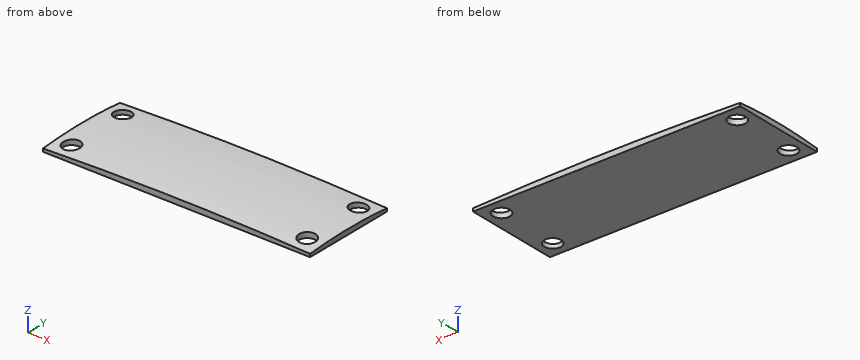
from build123d import *

# Parameters (mm, degrees)
SKETCH1_OUTSIDE_W       = 3552.458
SKETCH1_OUTSIDE_H       = 1860.818
SKETCH1_OUTSIDE_W_2     = 107.95
SKETCH1_OUTSIDE_H_2     = 38.1
CUT_EXTRUDE1_DEPTH      = 3115.745878548
CUT_EXTRUDE2_START      = -3.175
SKETCH3_W               = 107.95
SKETCH3_H               = 44.752430816
CUT_EXTRUDE2_DEPTH      = 2744.161532781
CUT_EXTRUDE3_DEPTH      = 58.326117654
CUT_EXTRUDE3_DEPTH_BACK = 58.326117654
SKETCH4_R               = 3.429


with BuildPart() as part:
    # Sketch2 → Revolve1 (revolve)
    with BuildSketch(Plane(origin=(0, 0, 0), x_dir=(0, 0, -1), z_dir=(1, 0, 0))):
        with BuildLine():
            Line((1372.87, -527.05), (1372.87, 527.05))
            add(Edge.make_bspline(
                [(1372.87, 527.05), (0, 527.05), (0, 0), (0, -527.05), (1372.87, -527.05)],
                knots=[4.71238898, 4.71238898, 4.71238898, 6.283185307, 6.283185307, 7.853981634, 7.853981634, 7.853981634], degree=2, weights=[1, 0.707106781, 1, 0.707106781, 1]))
        make_face()
    revolve(axis=Axis((0, -527.05, -1372.87), (0, 1, 0)))

    # Sketch1 outside → Cut-Extrude1 (cut, through all)
    with BuildSketch(Plane.XY):
        Rectangle(SKETCH1_OUTSIDE_W, SKETCH1_OUTSIDE_H)
        Rectangle(SKETCH1_OUTSIDE_W_2, SKETCH1_OUTSIDE_H_2, mode=Mode.SUBTRACT)
    extrude(amount=-CUT_EXTRUDE1_DEPTH, mode=Mode.SUBTRACT)

    # Sketch3 → Cut-Extrude2 (cut, through all)
    with BuildSketch(Plane.XY.offset(CUT_EXTRUDE2_START)):
        Rectangle(SKETCH3_W, SKETCH3_H)
    extrude(amount=-CUT_EXTRUDE2_DEPTH, mode=Mode.SUBTRACT)

    # Sketch4 → Cut-Extrude3 (cut, two sides: drawn at the far end of the back side and taken through both)
    with BuildSketch(Plane(origin=(0, 0, -3.175), x_dir=(-1, 0, 0), z_dir=(0, 0, -1)).offset(-CUT_EXTRUDE3_DEPTH_BACK)):
        with Locations((-47.625, -12.7)):
            Circle(SKETCH4_R)
        with Locations((-47.625, 12.7)):
            Circle(SKETCH4_R)
        with Locations((47.625, 12.7)):
            Circle(SKETCH4_R)
        with Locations((47.625, -12.7)):
            Circle(SKETCH4_R)
    extrude(amount=CUT_EXTRUDE3_DEPTH + CUT_EXTRUDE3_DEPTH_BACK, mode=Mode.SUBTRACT)


solid = part.part
Could you check a few things on this model? Use its own coordinates, in mm. Coordinates: 2 decimals unless noted, no trailing zeros. Loops run counter-clockwise (first coordinate to the right, second up) from the corner with the lowest first, then second, coordinate; pieces in that order, holes last. Notation, with made-up numbers: (-23, -5) -> (-17, -5) arc R23 ccw to (-17, 27) -> close; hole circle Ø2 at (5.5, 86.5). An arc over 180 degrees is marked (long way). Answer in a Markdown table with one row per item.
(1) Imagine slicing it at B-B (y = -12.7). Give the number of separate pieces and of enclosed holes in the cut face, plus the area to 3 significant figures.
Results found:
| item | result |
|---|---|
| separate pieces | 3 |
| enclosed holes | 0 |
| area | 235 mm^2 |
(2) If I drill on probe 1 along X at (y, z) = (-12.7, -2.4) (3 decimals); probe 2 along Y at (x, z) = (48, -2.75); probe 3 along X at (y, z) = (-15, -1.85) (3 decimals), over which ranges is the centre line in solid material (lowest first)?
Results found:
| item | result |
|---|---|
| probe 1 | x = -53.975 to -51.054, -44.196 to 44.196, 51.054 to 53.975 |
| probe 2 | y = -19.05 to -16.11, -9.29 to 9.29, 16.11 to 19.05 |
| probe 3 | x = -53.975 to -50.168, -45.082 to 45.082, 50.168 to 53.975 |
(3) Imagine slicing it at A-A (z = -2.6). List the corners of the cut face in (x, y) for me (3 decimals).
Results found:
| item | result |
|---|---|
| outline | (-53.975, -19.05) -> (53.975, -19.05) -> (53.975, 19.05) -> (-53.975, 19.05) -> close; hole circle Ø6.858 at (-47.625, -12.7); hole circle Ø6.858 at (-47.625, 12.7); hole circle Ø6.858 at (47.625, -12.7); hole circle Ø6.858 at (47.625, 12.7) |
(4) Will these pins go through, and if not, where does the flat tip stop? pin 1 Ø8 at (x, y) = (-29, -14.5) entering from +Z; pin 2 Ø5.5 at (x, y) = (-47.625, -12.7) entering from +Z; pin 3 Ø2 at (x, y) = (35.5, 12.5) entering from +Z; pin 4 Ø8 at (x, y) = (13.5, 0) entering from +Z.
Results found:
| item | result |
|---|---|
| pin 1 | stops at z = -0.56 |
| pin 2 | passes through |
| pin 3 | stops at z = -0.78 |
| pin 4 | stops at z = -0.03 |
